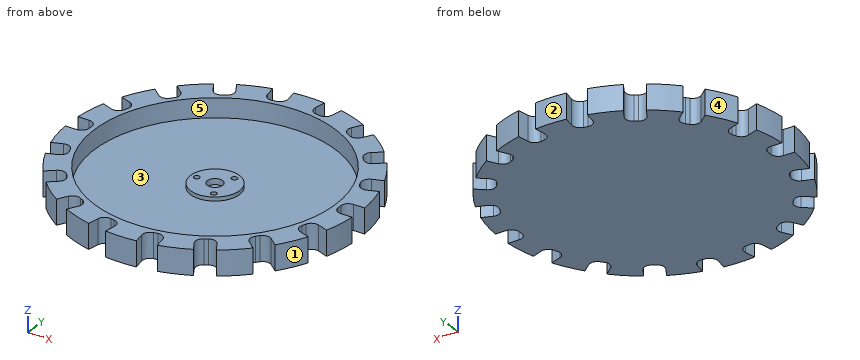
from build123d import *

# Parameters (mm, degrees)
F0_R     = 62.5
F0_R_2   = 12.7
F0_R_3   = 1.5
F0_R_4   = 4
F1_DEPTH = 3
F2_DEPTH = 13
F3_DEPTH = 5
F4_DEPTH = 2


with BuildPart() as f1:
    # F0 (on Top) → F1 (new body)
    with BuildSketch(Plane.XY):
        Circle(F0_R)
        Circle(F0_R_2, mode=Mode.SUBTRACT)
        Circle(F0_R_2)
        with Locations((-4.75, -8.227241)):
            Circle(F0_R_3, mode=Mode.SUBTRACT)
        with Locations((4.75, -8.227241)):
            Circle(F0_R_3, mode=Mode.SUBTRACT)
        with Locations((-9.5, 0)):
            Circle(F0_R_3, mode=Mode.SUBTRACT)
        with Locations((-4.75, 8.227241)):
            Circle(F0_R_3, mode=Mode.SUBTRACT)
        Circle(F0_R_4, mode=Mode.SUBTRACT)
        with Locations((4.75, 8.227241)):
            Circle(F0_R_3, mode=Mode.SUBTRACT)
        with Locations((9.5, 0)):
            Circle(F0_R_3, mode=Mode.SUBTRACT)
        with Locations((9.5, 0)):
            Circle(F0_R_3)
        with Locations((4.75, 8.227241)):
            Circle(F0_R_3)
        with Locations((-4.75, 8.227241)):
            Circle(F0_R_3)
        with Locations((-9.5, 0)):
            Circle(F0_R_3)
        with Locations((-4.75, -8.227241)):
            Circle(F0_R_3)
        with Locations((4.75, -8.227241)):
            Circle(F0_R_3)
    extrude(amount=F1_DEPTH)

    # F0 (on Top) → F2 (join)
    with BuildSketch(Plane.XY):
        with BuildLine():
            Line((69, 5), (74.833148, 5))
            ThreePointArc((74.833148, 5), (73.860581, 13.023613), (72.030257, 20.895981))
            Line((72.030257, 20.895981), (66.548892, 18.900927))
            ThreePointArc((66.548892, 18.900927), (63.490338, 19.034466), (61.42204, 21.291617))
            Line((61.42204, 21.291617), (60.738, 23.171002))
            ThreePointArc((60.738, 23.171002), (60.87154, 26.229556), (63.12869, 28.297853))
            Line((63.12869, 28.297853), (68.610056, 30.292907))
            ThreePointArc((68.610056, 30.292907), (64.951905, 37.5), (60.539455, 44.271598))
            Line((60.539455, 44.271598), (56.071005, 40.522123))
            ThreePointArc((56.071005, 40.522123), (53.151231, 39.601522), (50.435676, 41.01515))
            Line((50.435676, 41.01515), (49.150101, 42.547239))
            ThreePointArc((49.150101, 42.547239), (48.2295, 45.467012), (49.643129, 48.182567))
            Line((49.643129, 48.182567), (54.111579, 51.932042))
            ThreePointArc((54.111579, 51.932042), (48.209071, 57.453333), (41.746701, 62.307407))
            Line((41.746701, 62.307407), (38.830127, 57.255753))
            ThreePointArc((38.830127, 57.255753), (36.401302, 55.39205), (33.366025, 55.791651))
            Line((33.366025, 55.791651), (31.633975, 56.791651))
            ThreePointArc((31.633975, 56.791651), (29.770271, 59.220477), (30.169873, 62.255753))
            Line((30.169873, 62.255753), (33.086447, 67.307407))
            ThreePointArc((33.086447, 67.307407), (25.651511, 70.476947), (17.918678, 72.828023))
            Line((17.918678, 72.828023), (16.905763, 67.083494))
            ThreePointArc((16.905763, 67.083494), (15.260838, 64.501479), (12.271939, 63.838856))
            Line((12.271939, 63.838856), (10.302324, 64.186152))
            ThreePointArc((10.302324, 64.186152), (7.720308, 65.831077), (7.057685, 68.819976))
            Line((7.057685, 68.819976), (8.070601, 74.564505))
            ThreePointArc((8.070601, 74.564505), (0, 75), (-8.070601, 74.564505))
            Line((-8.070601, 74.564505), (-7.057685, 68.819976))
            ThreePointArc((-7.057685, 68.819976), (-7.720308, 65.831077), (-10.302324, 64.186152))
            Line((-10.302324, 64.186152), (-12.271939, 63.838856))
            ThreePointArc((-12.271939, 63.838856), (-15.260838, 64.501479), (-16.905763, 67.083494))
            Line((-16.905763, 67.083494), (-17.918678, 72.828023))
            ThreePointArc((-17.918678, 72.828023), (-25.651511, 70.476947), (-33.086447, 67.307407))
            Line((-33.086447, 67.307407), (-30.169873, 62.255753))
            ThreePointArc((-30.169873, 62.255753), (-29.770271, 59.220477), (-31.633975, 56.791651))
            Line((-31.633975, 56.791651), (-33.366025, 55.791651))
            ThreePointArc((-33.366025, 55.791651), (-36.401302, 55.39205), (-38.830127, 57.255753))
            Line((-38.830127, 57.255753), (-41.746701, 62.307407))
            ThreePointArc((-41.746701, 62.307407), (-48.209071, 57.453333), (-54.111579, 51.932042))
            Line((-54.111579, 51.932042), (-49.643129, 48.182567))
            ThreePointArc((-49.643129, 48.182567), (-48.2295, 45.467012), (-49.150101, 42.547239))
            Line((-49.150101, 42.547239), (-50.435676, 41.01515))
            ThreePointArc((-50.435676, 41.01515), (-53.151231, 39.601522), (-56.071005, 40.522123))
            Line((-56.071005, 40.522123), (-60.539455, 44.271598))
            ThreePointArc((-60.539455, 44.271598), (-64.951905, 37.5), (-68.610056, 30.292907))
            Line((-68.610056, 30.292907), (-63.12869, 28.297853))
            ThreePointArc((-63.12869, 28.297853), (-60.87154, 26.229556), (-60.738, 23.171002))
            Line((-60.738, 23.171002), (-61.42204, 21.291617))
            ThreePointArc((-61.42204, 21.291617), (-63.490338, 19.034466), (-66.548892, 18.900927))
            Line((-66.548892, 18.900927), (-72.030257, 20.895981))
            ThreePointArc((-72.030257, 20.895981), (-73.860581, 13.023613), (-74.833148, 5))
            Line((-74.833148, 5), (-69, 5))
            ThreePointArc((-69, 5), (-66.171573, 3.828427), (-65, 1))
            Line((-65, 1), (-65, -1))
            ThreePointArc((-65, -1), (-66.171573, -3.828427), (-69, -5))
            Line((-69, -5), (-74.833148, -5))
            ThreePointArc((-74.833148, -5), (-73.860581, -13.023613), (-72.030257, -20.895981))
            Line((-72.030257, -20.895981), (-66.548892, -18.900927))
            ThreePointArc((-66.548892, -18.900927), (-63.490338, -19.034466), (-61.42204, -21.291617))
            Line((-61.42204, -21.291617), (-60.738, -23.171002))
            ThreePointArc((-60.738, -23.171002), (-60.87154, -26.229556), (-63.12869, -28.297853))
            Line((-63.12869, -28.297853), (-68.610056, -30.292907))
            ThreePointArc((-68.610056, -30.292907), (-64.951905, -37.5), (-60.539455, -44.271598))
            Line((-60.539455, -44.271598), (-56.071005, -40.522123))
            ThreePointArc((-56.071005, -40.522123), (-53.151231, -39.601522), (-50.435676, -41.01515))
            Line((-50.435676, -41.01515), (-49.150101, -42.547239))
            ThreePointArc((-49.150101, -42.547239), (-48.2295, -45.467012), (-49.643129, -48.182567))
            Line((-49.643129, -48.182567), (-54.111579, -51.932042))
            ThreePointArc((-54.111579, -51.932042), (-48.209071, -57.453333), (-41.746701, -62.307407))
            Line((-41.746701, -62.307407), (-38.830127, -57.255753))
            ThreePointArc((-38.830127, -57.255753), (-36.401302, -55.39205), (-33.366025, -55.791651))
            Line((-33.366025, -55.791651), (-31.633975, -56.791651))
            ThreePointArc((-31.633975, -56.791651), (-29.770271, -59.220477), (-30.169873, -62.255753))
            Line((-30.169873, -62.255753), (-33.086447, -67.307407))
            ThreePointArc((-33.086447, -67.307407), (-25.651511, -70.476947), (-17.918678, -72.828023))
            Line((-17.918678, -72.828023), (-16.905763, -67.083494))
            ThreePointArc((-16.905763, -67.083494), (-15.260838, -64.501479), (-12.271939, -63.838856))
            Line((-12.271939, -63.838856), (-10.302324, -64.186152))
            ThreePointArc((-10.302324, -64.186152), (-7.720308, -65.831077), (-7.057685, -68.819976))
            Line((-7.057685, -68.819976), (-8.070601, -74.564505))
            ThreePointArc((-8.070601, -74.564505), (0, -75), (8.070601, -74.564505))
            Line((8.070601, -74.564505), (7.057685, -68.819976))
            ThreePointArc((7.057685, -68.819976), (7.720308, -65.831077), (10.302324, -64.186152))
            Line((10.302324, -64.186152), (12.271939, -63.838856))
            ThreePointArc((12.271939, -63.838856), (15.260838, -64.501479), (16.905763, -67.083494))
            Line((16.905763, -67.083494), (17.918678, -72.828023))
            ThreePointArc((17.918678, -72.828023), (25.651511, -70.476947), (33.086447, -67.307407))
            Line((33.086447, -67.307407), (30.169873, -62.255753))
            ThreePointArc((30.169873, -62.255753), (29.770271, -59.220477), (31.633975, -56.791651))
            Line((31.633975, -56.791651), (33.366025, -55.791651))
            ThreePointArc((33.366025, -55.791651), (36.401302, -55.39205), (38.830127, -57.255753))
            Line((38.830127, -57.255753), (41.746701, -62.307407))
            ThreePointArc((41.746701, -62.307407), (48.209071, -57.453333), (54.111579, -51.932042))
            Line((54.111579, -51.932042), (49.643129, -48.182567))
            ThreePointArc((49.643129, -48.182567), (48.2295, -45.467012), (49.150101, -42.547239))
            Line((49.150101, -42.547239), (50.435676, -41.01515))
            ThreePointArc((50.435676, -41.01515), (53.151231, -39.601522), (56.071005, -40.522123))
            Line((56.071005, -40.522123), (60.539455, -44.271598))
            ThreePointArc((60.539455, -44.271598), (64.951905, -37.5), (68.610056, -30.292907))
            Line((68.610056, -30.292907), (63.12869, -28.297853))
            ThreePointArc((63.12869, -28.297853), (60.87154, -26.229556), (60.738, -23.171002))
            Line((60.738, -23.171002), (61.42204, -21.291617))
            ThreePointArc((61.42204, -21.291617), (63.490338, -19.034466), (66.548892, -18.900927))
            Line((66.548892, -18.900927), (72.030257, -20.895981))
            ThreePointArc((72.030257, -20.895981), (73.860581, -13.023613), (74.833148, -5))
            Line((74.833148, -5), (69, -5))
            ThreePointArc((69, -5), (66.171573, -3.828427), (65, -1))
            Line((65, -1), (65, 1))
            ThreePointArc((65, 1), (66.171573, 3.828427), (69, 5))
        make_face()
        Circle(F0_R, mode=Mode.SUBTRACT)
    extrude(amount=F2_DEPTH)

    # F0 (on Top) → F3 (join)
    with BuildSketch(Plane.XY):
        Circle(F0_R_2)
        with Locations((-4.75, -8.227241)):
            Circle(F0_R_3, mode=Mode.SUBTRACT)
        with Locations((4.75, -8.227241)):
            Circle(F0_R_3, mode=Mode.SUBTRACT)
        with Locations((-9.5, 0)):
            Circle(F0_R_3, mode=Mode.SUBTRACT)
        with Locations((-4.75, 8.227241)):
            Circle(F0_R_3, mode=Mode.SUBTRACT)
        Circle(F0_R_4, mode=Mode.SUBTRACT)
        with Locations((4.75, 8.227241)):
            Circle(F0_R_3, mode=Mode.SUBTRACT)
        with Locations((9.5, 0)):
            Circle(F0_R_3, mode=Mode.SUBTRACT)
        with Locations((-4.75, 8.227241)):
            Circle(F0_R_3)
        with Locations((9.5, 0)):
            Circle(F0_R_3)
        with Locations((-4.75, -8.227241)):
            Circle(F0_R_3)
    extrude(amount=F3_DEPTH)

    # F0 (on Top) → F4 (join)
    with BuildSketch(Plane.XY):
        Circle(F0_R_4)
    extrude(amount=F4_DEPTH)


solid = f1.part
Work out the finished part from the listing and answer in its coordinate system (mm). Face numbers are marked on the shaded views. A direction names the side the tool comes from. Coordinates: 2 decimals unless noted, no trailing zeros. Loops run counter-clockwise (first coordinate to the right, second up) from the corner with the lowest first, then second, coordinate; pieces in that order, holes last. Notation, with made-up numbers: (9.25, -12.75) -> (64.25, -12.75) arc R14 ccw to (64.25, -8.75) -> close; hole circle Ø10 at (10.5, -36.75). An arc over 180 degrees is marked (long way). Write each question's results on one line, items separated by ' | '. Start each with the question number.
1) Consider line 1 along Y through (x, z) = (-9.5, 3.6); line 2 along Y through (x, z) = (4.75, 3.9); line 3 along X through (y, z) = (65.5, 7.5). Determine where each line is inside the solid, lowest interval first.
2) The mould has two halves that part along Y. Classify the marked faces 1, 2 and 3: pulls with the +Y half, pulls with the -Y half, needs draft (parallel to the pull), parting line crosses it, or undercut.
3) Find section A-A on x = 0. Determine the outline of the cut face in (y, z).
4) Flat-ended cylindrical pins translate along their axes: P1, Ø7.5, axis at x = -5.5, y = -0.5, coming from the +Z side; P2, Ø0.6, axis at y = -0.5, z = 8, coming from the +X side; P3, Ø2, axis at y = -17, z = 9.5, coming from the +X side. Find the tip coordinate at first contact, or state that the pin passes through.
5) For the marked faces 4 and 5, determine the directions among +Z, -Z, +X, -X, +Y, -Y from which every point of the face is accessible in a straight line to the end or side of a thin tool.
6) Find section B-B on x = -46.5. Determine the outline of the cut face in (y, z).
Response values:
1) line 1: y = -64.42 to -61.77, -8.43 to -1.5, 1.5 to 8.43, 61.77 to 64.42 | line 2: y = -74.85 to -62.32, -11.78 to -9.73, -6.73 to 6.73, 9.73 to 11.78, 62.32 to 74.85 | line 3: x = -32.04 to -16.25, -7.98 to 7.98, 16.25 to 32.04
2) face 1: pulls with the -Y half | face 2: pulls with the +Y half | face 3: undercut
3) outline: (-75, 0) -> (75, 0) -> (75, 13) -> (62.5, 13) -> (62.5, 3) -> (12.7, 3) -> (12.7, 5) -> (4, 5) -> (4, 2) -> (-4, 2) -> (-4, 5) -> (-12.7, 5) -> (-12.7, 3) -> (-62.5, 3) -> (-62.5, 13) -> (-75, 13) -> close
4) P1: stops at z = 5 | P2: stops at x = 65 | P3: stops at x = 73.27
5) face 4: +Z, -Z, -X, +Y | face 5: +Z
6) outline: (-58.85, 0) -> (58.85, 0) -> (58.85, 13) -> (41.76, 13) -> (41.76, 3) -> (-41.76, 3) -> (-41.76, 13) -> (-58.85, 13) -> close
